```python
from build123d import *

# Parameters (mm, degrees)
F0_W     = 30
F0_H     = 60
F1_DEPTH = 5
F2_R     = 4.75
F2_R_2   = 4.6875
F2_R_3   = 4.625
F2_R_4   = 4.5625
F2_R_5   = 2
F2_R_6   = 2.0625
F2_R_7   = 2.125
F2_R_8   = 2.1875
F2_R_9   = 2.25
F3_DEPTH = 5.001


with BuildPart() as f1:
    # F0 (on Top) → F1 (new body)
    with BuildSketch(Plane.XY):
        with Locations((-5, 0)):
            Rectangle(F0_W, F0_H)
    extrude(amount=F1_DEPTH)

    # F2 (on face) → F3 (cut, through all)
    with BuildSketch(Plane.XY.offset(5)):
        with Locations((-10, 22.5)):
            Circle(F2_R)
        with Locations((-10, 7.5)):
            Circle(F2_R_2)
        with Locations((-10, -7.5)):
            Circle(F2_R_3)
        with Locations((-10, -22.5)):
            Circle(F2_R_4)
        with Locations((5, -20)):
            Circle(F2_R_5)
        with Locations((5, -10)):
            Circle(F2_R_6)
        with Locations((5, 0)):
            Circle(F2_R_7)
        with Locations((5, 10)):
            Circle(F2_R_8)
        with Locations((5, 20)):
            Circle(F2_R_9)
    extrude(amount=-F3_DEPTH, mode=Mode.SUBTRACT)


solid = f1.part
```
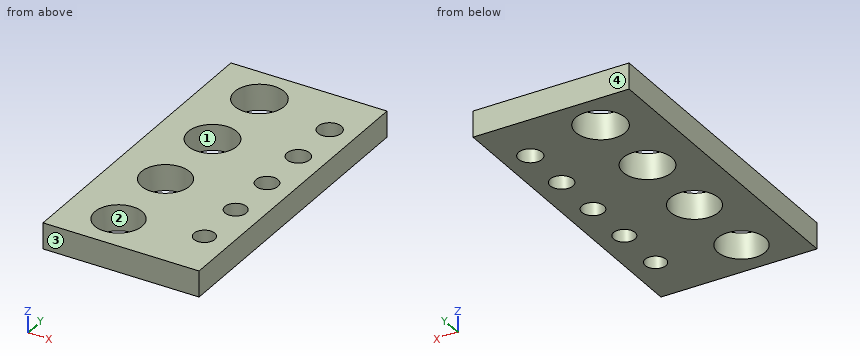
Part model, mm, in its own coordinate system. Face numbers are marked on the shaded views. Round coordinates to 2 decimals unless told otherwise and drop trailing zeros. Loops run counter-clockwise (first coordinate to the right, second up) from the corner with the lowest first, then second, coordinate; pieces in that order, holes last. Notation, with made-up numbers: (-27.75, -31.5) -> (-17.75, -31.5) arc R26 ccw to (-17.75, -10.5) -> close; hole circle Ø9 at (39.25, 16.5). An arc over 180 degrees is marked (long way). Use a Markdown table: item, result.
1) Drop flat-ended pins along their axis: pin 1 Ø8.5 at (x, y) = (-10, -7.5) entering from -Z; pin 2 Ø5.5 at (x, y) = (5, -10) entering from -Z. Give the stop position or say it passes through.
The answers:
| item | result |
|---|---|
| pin 1 | passes through |
| pin 2 | stops at z = 0 |
2) Pull direction Y, two halves, no side cores. Call the marked faces 1, 2, 3 and 4: pulls with the +Y half, pulls with the -Y half, needs draft (parallel to the pull), parting line crosses it, or undercut.
The answers:
| item | result |
|---|---|
| face 1 | undercut |
| face 2 | undercut |
| face 3 | pulls with the -Y half |
| face 4 | pulls with the +Y half |
3) Probe line 1 (Y direction, x = -13, z = 3.7); line 2 (Y direction, x = -10.5, z = 2.85); line 3 (X direction, y = -10.5, z = 3.15). List the from-to ranges inside material, lowest first. Write a range as [from, to].
The answers:
| item | result |
|---|---|
| line 1 | y = [-30, -25.94], [-19.06, -11.02], [-3.98, 3.9], [11.1, 18.82], [26.18, 30] |
| line 2 | y = [-30, -27.04], [-17.96, -12.1], [-2.9, 2.84], [12.16, 17.78], [27.22, 30] |
| line 3 | x = [-20, -13.52], [-6.48, 3], [7, 10] |
4) Cut at C-C, the plane y = 20. List the corners of the cut face in (x, z), and give its area (3 significant figures).
The answers:
| item | result |
|---|---|
| outline | (-20, 0) -> (-14.04, 0) -> (-14.04, 5) -> (-20, 5) -> close; (-5.96, 0) -> (2.75, 0) -> (2.75, 5) -> (-5.96, 5) -> close; (7.25, 0) -> (10, 0) -> (10, 5) -> (7.25, 5) -> close |
| area | 87.1 mm2 |
5) Cut at A-A, the plane x = 5. State how many separate pieces and enclosed holes the cut face has, and give its area (3 significant figures).
The answers:
| item | result |
|---|---|
| separate pieces | 6 |
| enclosed holes | 0 |
| area | 194 mm2 |
